Here's how the part is built. I have some questions about the finished solid (model axes, mm). A direction names the side the tool comes from. Give positions to 0.01 mm unless a question says otherwise; leave off trailing zeros. Write each loop counter-clockwise with the first axis right and the second up, starting at its lowest first coordinate (ties: lowest second). Pieces come first, ordered by that corner, then holes. Notation, with made-up numbers: (-18, 41.5) -> (29, 41.5) arc R35 ccw to (29, 74.5) -> close; hole circle Ø1 at (-38.75, 9). An arc over 180 degrees is marked (long way). Return JSON: item names as keys, results as strings.
from build123d import *

# Parameters (mm, degrees)
SKETCH2_R                = 5
SKETCH2_R_2              = 3
BOSS_EXTRUDE1_DEPTH      = 12
BOSS_EXTRUDE1_DEPTH_BACK = 12
SKETCH3_R                = 20
SKETCH4_R                = 10
CUT_EXTRUDE1_DEPTH       = 32


with BuildPart() as part:
    # Sweep1: sweep along a path in Sketch1
    with BuildLine(Plane.XY) as sweep1_path:
        ThreePointArc((-267, -267), (0, 0), (267, -267))
    # Sketch2 → Sweep1 (sweep)
    with BuildSketch(Plane(origin=(0, 0, 0), x_dir=(0, 0, -1), z_dir=(1, 0, 0))):
        Circle(SKETCH2_R)
        Circle(SKETCH2_R_2, mode=Mode.SUBTRACT)
    sweep(path=sweep1_path.line)

    # Sketch3 → Boss-Extrude1 (add, two sides: drawn at the far end of the back side and taken through both)
    with BuildSketch(Plane(origin=(0, 0, 0), x_dir=(1, 0, 0), z_dir=(0, 1, 0)).offset(-BOSS_EXTRUDE1_DEPTH_BACK)):
        with Locations(Location((0, 0, 0), (0, 0, 270))):
            Circle(SKETCH3_R)
    extrude(amount=BOSS_EXTRUDE1_DEPTH + BOSS_EXTRUDE1_DEPTH_BACK)

    # Sketch4 → Cut-Extrude1 (cut)
    with BuildSketch(Plane(origin=(0, 12, 0), x_dir=(1, 0, 0), z_dir=(0, 1, 0))):
        with Locations(Location((0, 0, 0), (0, 0, 270))):
            Circle(SKETCH4_R)
    extrude(amount=-CUT_EXTRUDE1_DEPTH, mode=Mode.SUBTRACT)


solid = part.part
1. Suppose I cut it at B-B, the plane y = -157. Count the separate pieces of the cut face and the enclosed holes in it, and give its area (3 significant figures).
Taken from the geometry:
{"separate pieces": "2", "enclosed holes": "2", "area": "110 mm²"}
2. For pin 1 Ø12 at (x, z) = (108, -8) entering from -Y; pin 2 Ø8 at (x, z) = (-126, 6.5) entering from -Y; pin 3 Ø12 at (y, z) = (-235, -4.5) entering from +X, each with a flat end and sliding along its axis, tell me the tip position at first contact or that it passes through.
Taken from the geometry:
{"pin 1": "stops at y = -28.73", "pin 2": "stops at y = -37.22", "pin 3": "stops at x = 270.58"}
3. Suppose I cut it at A-A, the plane x = 0. List the corners of the cut face in (y, z) for me.
Taken from the geometry:
{"outline": "(-12, -20) -> (12, -20) -> (12, -10) -> (-12, -10) -> close; (-12, 10) -> (12, 10) -> (12, 20) -> (-12, 20) -> close"}
4. Which directions (+Z, -Z, +X, -X, +Y, -Y) give clear straight access to the entire face, cutting with the end or side of a thin tool? Please do faces 1 (the face through (9, -12, -5)), 2 (the face through (-270.3, -267, -0.1)).
Taken from the geometry:
{"face 1": "+Z, -Z, -Y", "face 2": "+Z, -Z, +X, -X, -Y"}
5. If I drill on line 1 (X direction, y = 7, z = 0); line 2 (Y direction, x = -1.5, z = -13.5); line 3 (Y direction, x = 80, z = -1.5), over which ranges is the centre line in solid material (lowest first)? Write a range as [from, to].
Taken from the geometry:
{"line 1": "x = [-20, -10], [10, 20]", "line 2": "y = [-12, 12]", "line 3": "y = [-17.27, -14.99], [-9.54, -7.27]"}
6. If we mould it in two halves opening along Z, with no side actions, what happens to faces 3 (the face through (-17.743, -0.168, 9.229)), 4 (the face through (-9.76, 0.17, -2.17)), 5 (the face through (9, 12, -5))? For each: released by +Z, released by -Z, zero draft, split by the parting line, or undercut.
Taken from the geometry:
{"face 3": "split by the parting line", "face 4": "undercut", "face 5": "zero draft"}
